```python
from build123d import *

# Parameters (mm, degrees)
F0_R     = 21.1
F0_R_2   = 19.1
F1_DEPTH = 600
F4_D     = 6.5
F4_DEPTH = 10


with BuildPart() as f1:
    # F0 (on Right) → F1 (new body, symmetric)
    with BuildSketch(Plane.YZ):
        Circle(F0_R)
        Circle(F0_R_2, mode=Mode.SUBTRACT)
    extrude(amount=F1_DEPTH, both=True)

    # F4
    with Locations(Plane(origin=(0, 0, -25), x_dir=(1, 0, 0), z_dir=(0, 0, -1))):
        with Locations((-500, 0), (-457, 0), (457, 0), (500, 0)):
            Hole(F4_D / 2, depth=F4_DEPTH)


solid = f1.part
```
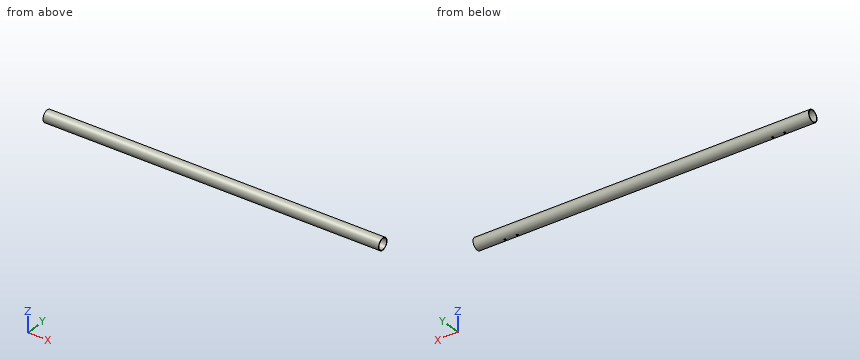
Check sheet for the modelled part. Datum: model origin and axes. Units: mm. Round coordinates to 2 decimals unless told otherwise and drop trailing zeros. Order: outer loops, then holes, each group sorted by start corner. A loop starts at its lowest first (then second) coordinate and runs counter-clockwise, first axis right, second up. Notation, with made-up numbers: (39, 74) - (75, 74) arc R16 cw to (75, 81) - close; hole circle Ø10 at (39, 52.25). An arc over 180 degrees is marked (long way). Write item = value, one per line.
Q1. Section check B-B (x = -331). Record the boundary of the cut face in (y, z), and give its area (3 significant figures).
Computed:
outline = circle Ø42.2 at (0, 0); hole circle Ø38.2 at (0, 0)
area = 253 mm^2
Q2. Section check A-A (z = 0). Record the boundary of the cut face in (x, y), and give its area (3 significant figures).
Computed:
outline = (-600, -21.1) - (600, -21.1) - (600, -19.1) - (-600, -19.1) - close; (-600, 19.1) - (600, 19.1) - (600, 21.1) - (-600, 21.1) - close
area = 4,800 mm^2
Q3. Thickness scan on line 1 along Z through (x, y) = (-300.5, 1); line 2 along Z through (x, y) = (19, -2) (3 decimals); line 3 along Y through (x, z) = (457, -19). Record the ranges inside material, lowest first.
Computed:
line_1 = -21.08 to -19.07, 19.07 to 21.08
line_2 = -21.005 to -18.995, 18.995 to 21.005
line_3 = -9.18 to -3.25, 3.25 to 9.18
Q4. Go/stop test with flat-tipped pins: pin 1 (5 mm diameter, centred on x = 172, z = 3.5, fed in from +Y); pin 2 (4 mm diameter, centred on x = 457, y = 0, fed in from -Z) (3 decimals); pin 3 (6 mm diameter, centred on x = -403, y = 0.5, fed in from +Z). Record where each tip stops, or that it passes through.
Computed:
pin_1 = 21.08
pin_2 = 18.995
pin_3 = 21.1
